The listing builds one solid part. Answer for the finished solid, in the listing's coordinates (mm). Face numbers are marked on the shaded views. A direction names the side the tool comes from. Give positions to 0.01 mm unless a question says otherwise; leave off trailing zeros. Loops run counter-clockwise (first coordinate to the right, second up) from the corner with the lowest first, then second, coordinate; pieces in that order, holes last. Notation, with made-up numbers: (-7.75, 85.25) - (9.25, 85.25) arc R31 ccw to (9.25, 116.25) - close; hole circle Ø3 at (67, 4.5). An arc over 180 degrees is marked (long way). Answer in a Markdown table with one row per item. Add a question column.
```python
from build123d import *

# Parameters (mm, degrees)
F1_DEPTH = 38.1
F2_DEPTH = 12.7
F3_D     = 22.225
F5_D     = 9.525
F6_D     = 9.525


with BuildPart() as f1:
    # F0 (on Front) → F1 (new body)
    with BuildSketch(Plane.XZ):
        Polygon((0, 9.525), (0, 0), (127, 0), (127, 9.525), (101.6, 9.525), align=None)
    extrude(amount=F1_DEPTH)

    # F0 (on Front) → F2 (join)
    with BuildSketch(Plane.XZ):
        with BuildLine():
            Line((89.0406588905, 60.1776572782), (0, 9.525))
            Line((0, 9.525), (101.6, 9.525))
            Line((101.6, 9.525), (127, 9.525))
            Line((127, 9.525), (126.7595108524, 34.6130222733))
            Line((126.7595108524, 34.6130222733), (126.6880426637, 42.0686414936))
            ThreePointArc((126.6880426637, 42.0686414936), (112.6102771914, 60.989600175), (89.0406588905, 60.1776572782))
        make_face()
    extrude(amount=F2_DEPTH)

    # F3 (through all)
    with Locations(Plane(origin=(0, 0, 0), x_dir=(1, 0, 0), z_dir=(0, 1, 0))):
        with Locations((101.6, -38.1)):
            Hole(F3_D / 2)

    # F5 (through all)
    with Locations(Plane.XY.offset(9.525)):
        with Locations((25.399999693, -25.4)):
            Hole(F5_D / 2)

    # F6 (through all)
    with Locations(Plane.XY.offset(9.525)):
        with Locations((101.6, -25.4)):
            Hole(F6_D / 2)


solid = f1.part
```
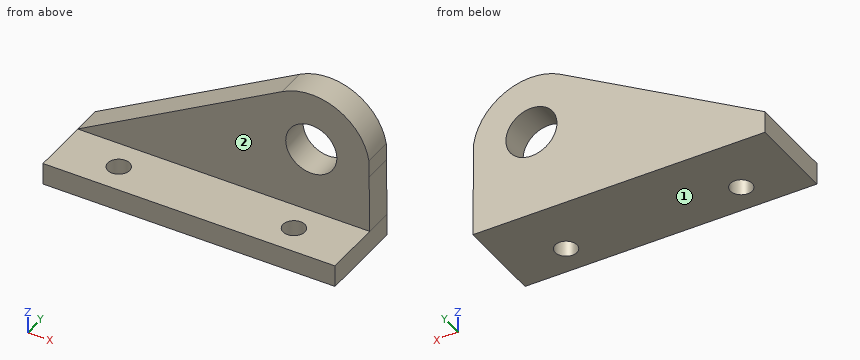
(1) Given pin 1 Ø20.5 at (x, y) = (44, -27.5) entering from +Z (3 decimals); pin 2 Ø3 at (x, z) = (64, 19.5) entering from -Y; pin 3 Ø1 at (x, y) = (41, -8.5) entering from +Z; pin 4 Ø4 at (x, y) = (84, -16.5) entering from -Z, each flat-ended and moving along its own axis, determine where each tip first touches the part or whether it passes through.
(2) A cutting plane is placed at C-C on z = 38.1. Determine the outline of the cut face in (x, y), plus the area to 3 significant figures.
(3) Find the intervals of material crossed by line 1 along Y through (x, z) = (101.6, 4.25); line 2 along X through (y, z) = (-22, 3); line 3 along Z through (x, y) = (75.5, -22.5) (3 decimals), in increasing order. Write a range as [from, to].
(4) A cutting plane is placed at D-D on y = -25.4. Determine the outline of the cut face in (x, z) (1 decimal), plus the area to 3 significant figures.
(5) A tool of negligible diameter and unlimited length cuts with its end or side. For the marked faces 1 and 2, from which of +Z, -Z, +X, -X, +Y, -Y can it reach the whole face along a straight path? Write none if from no direction.
(6) A cutting plane is placed at A-A on x = 101.6. Determine the outline of the cut face in (y, z) (1 decimal).
(7) A cutting plane is placed at B-B on y = -10. Determine the outline of the cut face in (x, z) (1 decimal), plus the area to 3 significant figures.
Evaluation:
| question | item | result |
|---|---|---|
| 1 | pin 1 | stops at z = 9.525 |
| 1 | pin 2 | stops at y = -12.7 |
| 1 | pin 3 | stops at z = 33.13 |
| 1 | pin 4 | stops at z = 0 |
| 2 | outline | (50.23, -12.7) - (90.49, -12.7) - (90.49, 0) - (50.23, 0) - close; (112.71, -12.7) - (126.73, -12.7) - (126.73, 0) - (112.71, 0) - close |
| 2 | area | 689 mm² |
| 3 | line 1 | y = [-38.1, -30.16], [-20.64, 0] |
| 3 | line 2 | x = [0, 22.07], [28.73, 98.27], [104.93, 127] |
| 3 | line 3 | z = [0, 9.525] |
| 4 | outline | (0, 0) - (20.6, 0) - (20.6, 9.5) - (0, 9.5) - close; (30.2, 0) - (96.8, 0) - (96.8, 9.5) - (30.2, 9.5) - close; (106.4, 0) - (127, 0) - (127, 9.5) - (106.4, 9.5) - close |
| 4 | area | 1,030 mm² |
| 5 | face 1 | -Z, +X, -X, +Y, -Y |
| 5 | face 2 | +Z, +X, -X, -Y |
| 6 | outline | (-38.1, 0) - (-30.2, 0) - (-30.2, 9.5) - (-38.1, 9.5) - close; (-20.6, 0) - (0, 0) - (0, 27) - (-12.7, 27) - (-12.7, 9.5) - (-20.6, 9.5) - close; (-12.7, 49.2) - (0, 49.2) - (0, 63.5) - (-12.7, 63.5) - close |
| 7 | outline | (0, 0) - (127, 0) - (127, 9.5) - (126.7, 42.1) arc R25.4 ccw to (89, 60.2) - (0, 9.5) - close; hole circle Ø22.2 at (101.6, 38.1) |
| 7 | area | 4,970 mm² |
